Autodesk Inventor part; units mm, degrees
ref_plane "YZ Plane" through (0, 0, 0) normal (1, 0, 0) x (0, 1, 0)
ref_plane "XZ Plane" through (0, 0, 0) normal (0, 1, 0) x (-1, 0, 0)
ref_plane "XY Plane" through (0, 0, 0) normal (0, 0, 1) x (1, 0, 0)
sketch "Sketch1" plane through (0, 0, 0) normal (0, 0, 1) x (1, 0, 0)
  line L0 (2.5, 0) -> (2.5, 9.4)
  line L1 (2.5, 9.4) -> (7, 9.4)
  line L2 (7, 9.4) -> (7, 8.2)
  line L3 (7, 8.2) -> (4.15, 8.2)
  line L4 (4.15, 8.2) -> (4.15, 1.2)
  line L5 (4.15, 1.2) -> (7, 1.2)
  line L6 (7, 1.2) -> (7, 0)
  line L7 (7, 0) -> (2.5, 0)
  line L8 (0, 0) -> (0, 3.2914)
  dimension "d0" = 2.5
  dimension "d2" = 9.4
  dimension "d3" = 1.2
  dimension "d4" = 1.2
  dimension "d5" = 7
  dimension "d6" = 4.15
revolve "Revolution1" add sketch "Sketch1" angle 360 about axis through (0, 0, 0) along (0, 1, 0)
properties part number "XcrLeftPulleyAlu"
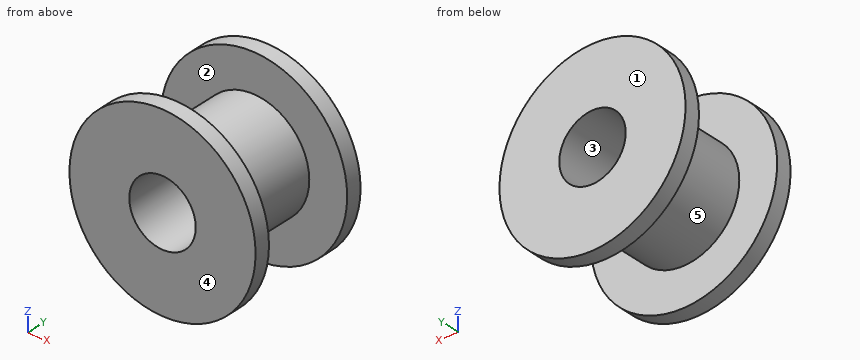
Source: CAD feature listing. Evaluate the final solid. Frame: model axes, mm. Face numbers are marked on the shaded views. A direction names the side the tool comes from. Give positions to 0.01 mm unless a question says otherwise; leave off trailing zeros. Loops run counter-clockwise (first coordinate to the right, second up) from the corner with the lowest first, then second, coordinate; pieces in that order, holes last. Notation, with made-up numbers: (-18.75, -8.75) - (7.25, -8.75) arc R22 ccw to (7.25, 27.25) - close; hole circle Ø5 at (11.5, 51). An arc over 180 degrees is marked (long way). Use CSV: the item, a comma, the result in double quotes.
1) Mould query, pull axis Z, two halves, no side actions, for the marked faces 3, 4 and 5. Classes: +Z half, -Z half, draft (parallel to the pull), parting line (faces both ways), or undercut.
Worked out:
face 3,"undercut"
face 4,"draft"
face 5,"parting line"
2) Cut plane C-C (y = 8.75). Output: boundary loops of the cut face in (x, z), and give its area (3 significant figures).
Worked out:
outline,"circle Ø14 at (0, 0); hole circle Ø5 at (0, 0)"
area,"134 mm^2"
3) Set-up query: the marked faces 1 and 2. Return all of +Z, -Z, +X, -X, +Y, -Y with unobstructed straight access to the full face (end or side cutting, diameter ignored); none if empty.
Worked out:
face 1,"+Z, -Z, +X, -X, +Y"
face 2,"none"
4) Cut plane D-D (x = 5.75). Output: boundary loops of the cut face in (y, z), and give its area (3 significant figures).
Worked out:
outline,"(0, -3.99) - (1.2, -3.99) - (1.2, 3.99) - (0, 3.99) - close; (8.2, -3.99) - (9.4, -3.99) - (9.4, 3.99) - (8.2, 3.99) - close"
area,"19.2 mm^2"
5) Pin query (flat end, axial travel): P1, Ø3, axis at y = 4, z = 1.5, coming from the +X side; P2, Ø2, axis at y = 1, z = 3.5, coming from the +X side. Return the tip coordinate at first contact, or that it passes through.
Worked out:
P1,"stops at x = 4.15"
P2,"stops at x = 6.54"
6) Cut plane A-A (z = 0). Output: boundary loops of the cut face in (x, y).
Worked out:
outline,"(-7, 0) - (-2.5, 0) - (-2.5, 9.4) - (-7, 9.4) - (-7, 8.2) - (-4.15, 8.2) - (-4.15, 1.2) - (-7, 1.2) - close; (2.5, 0) - (7, 0) - (7, 1.2) - (4.15, 1.2) - (4.15, 8.2) - (7, 8.2) - (7, 9.4) - (2.5, 9.4) - close"
7) Cut plane B-B (x = 0). Output: boundary loops of the cut face in (y, z), and give its area (3 significant figures).
Worked out:
outline,"(0, -7) - (1.2, -7) - (1.2, -4.15) - (8.2, -4.15) - (8.2, -7) - (9.4, -7) - (9.4, -2.5) - (0, -2.5) - close; (0, 2.5) - (9.4, 2.5) - (9.4, 7) - (8.2, 7) - (8.2, 4.15) - (1.2, 4.15) - (1.2, 7) - (0, 7) - close"
area,"44.7 mm^2"
8) Line query: line 1 (Y direction, x = 2, z = 5.75); line 2 (Z direction, x = 0, y = 2.5). Output: solid intervals per line, ascending.
Worked out:
line 1,"y = 0 to 1.2, 8.2 to 9.4"
line 2,"z = -4.15 to -2.5, 2.5 to 4.15"
